Autodesk Fusion 360 part; units mm, degrees
sketch "Sketch1" plane through (0, 0, 0) normal (0, 0, 1) x (1, 0, 0)
  circle A0 centre (74.5, 0) radius 2
  dimension "d1" = 4
  dimension "d2" = 74.5
revolve "Revolve1" add sketch "Sketch1" angle 360 about axis through (0, 1.75, 0) along (0, 1, 0)
equation "d2 = ( 145 / 2 ) * 1 mm + 2 mm"

Autodesk Fusion 360 part; units mm, degrees
sketch "Sketch1" plane through (0, 0, 0) normal (0, 0, 1) x (1, 0, 0)
  line L0 (45, 44.5) -> (45, -55.5)
  line L1 (45, -55.5) -> (47.5, -55.5)
  line L2 (47.5, -55.5) -> (47.5, -15.5)
  line L3 (47.5, -15.5) -> (57.5, -15.5)
  line L4 (57.5, -15.5) -> (57.5, 15.5)
  line L5 (57.5, 15.5) -> (47.5, 15.5)
  line L6 (47.5, 15.5) -> (47.5, 44.5)
  line L7 (47.5, 44.5) -> (45, 44.5)
  line L8 (0, 0) -> (57.5, 0) construction
  line L9 (45, 15.5) -> (42.5, 15.5)
  line L10 (42.5, 15.5) -> (42.5, -15.5)
  line L11 (42.5, -15.5) -> (45, -15.5)
  dimension "d1" = 45
  dimension "d2" = 47.5
  dimension "d4" = 31
  dimension "d8" = 29
  dimension "d9" = 40
  dimension "d10" = 100
  dimension "d11" = 57.5
  dimension "d12" = 42.5
revolve "Revolve1" add sketch "Sketch1" angle 360 about axis through (0, 1.75, 0) along (0, 1, 0)
equation "d1 = ( 90 / 2 ) * 1 mm"
equation "d2 = ( 95 / 2 ) * 1 mm"
equation "d11 = ( 115 / 2 ) * 1 mm"
equation "d12 = ( 85 / 2 ) * 1 mm"
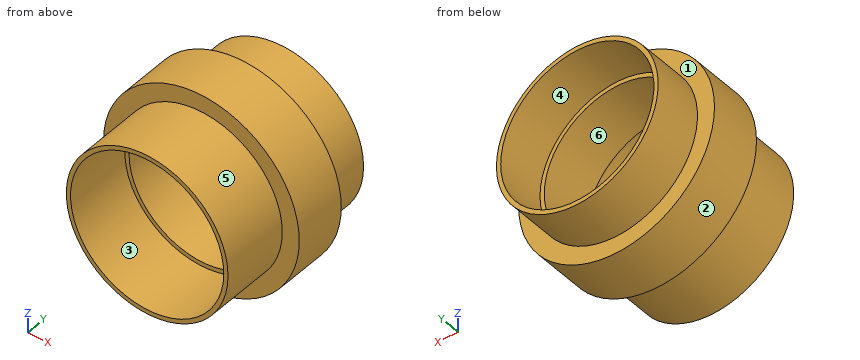
Verification items for the finished model (mm, model axes). Face numbers are marked on the shaded views. A direction names the side the tool comes from. Give positions to 0.01 mm unless a question says otherwise; leave off trailing zeros. Loops run counter-clockwise (first coordinate to the right, second up) from the corner with the lowest first, then second, coordinate; pieces in that order, holes last.
1. Cross-section at D-D on y = 34. Record the cut outline in (x, z).
Derived:
outline: circle Ø95 at (0, 0); hole circle Ø90 at (0, 0)
2. Tool access check on the marked faces 4, 5 and 6. Record the directions out of +Z, -Z, +X, -X, +Y, -Y that give a thin tool (end or side, any length) a straight path to the whole face; none if there is none.
Derived:
face 4: +Y
face 5: -Y
face 6: +Y, -Y
3. Go/stop test with flat-tipped pins: P1, Ø4, axis at x = -32, y = 7.5, coming from the -Z side; P2, Ø2, axis at y = -12, z = -40, coming from the +X side; P3, Ø1.5, axis at y = 26.5, z = 24.5, coming from the +X side. Record where each tip stops, or that it passes through.
Derived:
P1: stops at z = -49.05
P2: stops at x = 42.25
P3: stops at x = 41.14
4. Material ranges on probe 1 along Z at (x, y) = (0, -8.5); probe 2 along X at (y, z) = (27.5, 0), recorded low to high.
Derived:
probe 1: z = -57.5 to -42.5, 42.5 to 57.5
probe 2: x = -47.5 to -45, 45 to 47.5
5. Cross-section at B-B on x = 0. Record the cut outline in (y, z), and give its area (4 significant figures).
Derived:
outline: (-55.5, -47.5) - (-15.5, -47.5) - (-15.5, -57.5) - (15.5, -57.5) - (15.5, -47.5) - (44.5, -47.5) - (44.5, -45) - (15.5, -45) - (15.5, -42.5) - (-15.5, -42.5) - (-15.5, -45) - (-55.5, -45) - close; (-55.5, 45) - (-15.5, 45) - (-15.5, 42.5) - (15.5, 42.5) - (15.5, 45) - (44.5, 45) - (44.5, 47.5) - (15.5, 47.5) - (15.5, 57.5) - (-15.5, 57.5) - (-15.5, 47.5) - (-55.5, 47.5) - close
area: 1,275 mm2
6. Cross-section at A-A on z = 0. Record the cut outline in (x, y).
Derived:
outline: (-57.5, -15.5) - (-47.5, -15.5) - (-47.5, -55.5) - (-45, -55.5) - (-45, -15.5) - (-42.5, -15.5) - (-42.5, 15.5) - (-45, 15.5) - (-45, 44.5) - (-47.5, 44.5) - (-47.5, 15.5) - (-57.5, 15.5) - close; (42.5, -15.5) - (45, -15.5) - (45, -55.5) - (47.5, -55.5) - (47.5, -15.5) - (57.5, -15.5) - (57.5, 15.5) - (47.5, 15.5) - (47.5, 44.5) - (45, 44.5) - (45, 15.5) - (42.5, 15.5) - close
7. Release check for a two-part mould opening along Z. For the marked faces 1, 2 and 3 record: +Z half, -Z half, draft (parallel to the pull), parting line (faces both ways), or undercut.
Derived:
face 1: draft
face 2: parting line
face 3: undercut
8. Cross-section at C-C on y = 13.5. Record the cut outline in (x, z).
Derived:
outline: circle Ø115 at (0, 0); hole circle Ø85 at (0, 0)
